Design review of the part shown in the three views and the two pictorial views. Dimensions are in mm from the part's minimum x, y and z. Coordinates: 2 decimals unless noted, no trailing zeros. Write each loop counter-clockwise with the first axis right and the second up, starting at its lowest first coordinate (ties: lowest second). Pieces come first, ordered by that corner, then holes. Notation, with made-up numbers: M -10.75,30.25 L 24.25,30.25 A17 cw 24.25,35.25 Z; hole C -6,63 d8. An arc over 180 degrees is marked long. Answer as a JSON object with one key per item and string values.
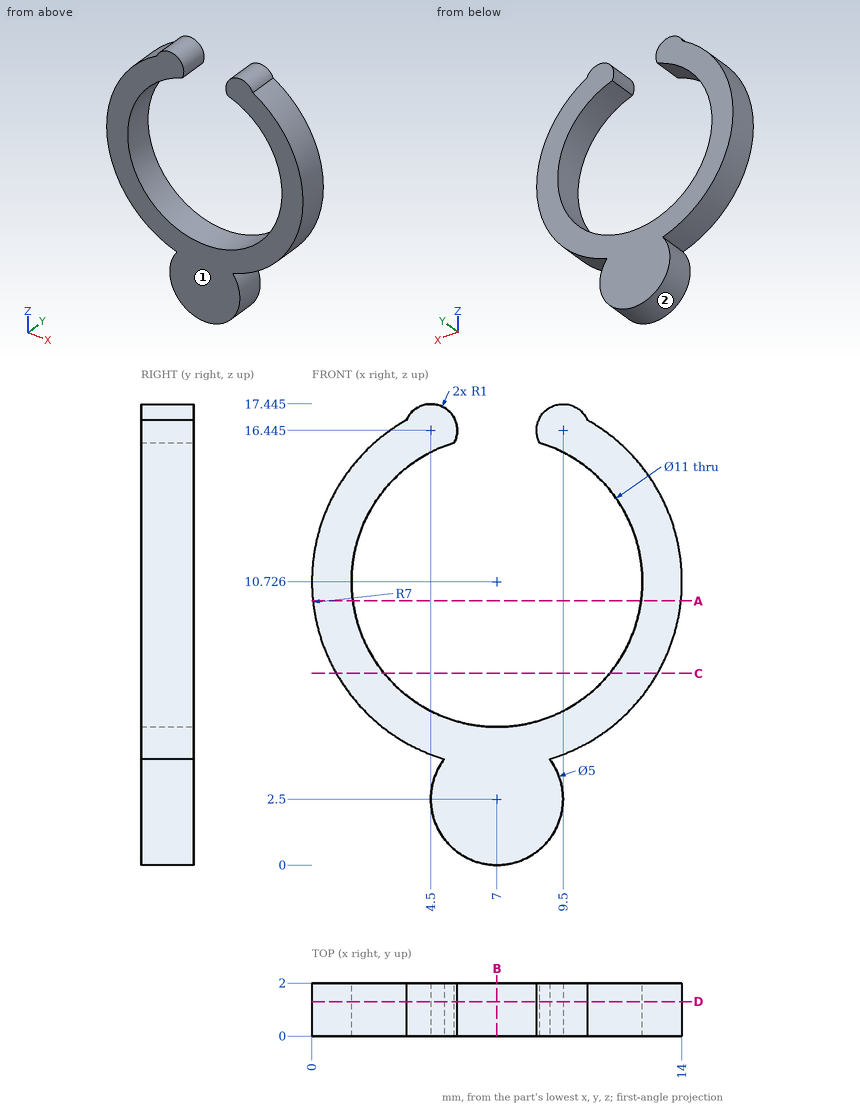
(1) Add section A-A on z = 10. Give the boundary of the cut face in (x, y).
Results list:
{"outline": "M 0.04,0 L 1.55,0 L 1.55,2 L 0.04,2 Z; M 12.45,0 L 13.96,0 L 13.96,2 L 12.45,2 Z"}
(2) For pin 1 Ø1 at (y, z) = (1.5, 6.5) entering from -X (1 decimal); pin 2 Ø8 at (x, z) = (12, 15.5) entering from -Y, all flat-tipped, find the tip position at first contact; note any pin that passes through.
Results list:
{"pin 1": "x = 1.1", "pin 2": "y = 0"}
(3) Draft analysis for pull direction Z (two halves, no side actions). For the marked faces 1 and 2, state which applies: released by +Z, released by -Z, zero draft, split by the parting line, or undercut.
Results list:
{"face 1": "zero draft", "face 2": "undercut"}
(4) Add section D-D on y = 1.3. Give the boundary of the cut face in (x, z) (1 decimal).
Results list:
{"outline": "M 3.6,16.8 A7 ccw 5,4 A2.5 ccw long 9,4 A7 ccw 10.4,16.8 A1 ccw long 8.6,16 A5.5 cw long 5.4,16 A1 ccw long Z"}
(5) Add section C-C on z = 7.25. Give the boundary of the cut face in (x, y).
Results list:
{"outline": "M 0.92,0 L 2.74,0 L 2.74,2 L 0.92,2 Z; M 11.26,0 L 13.08,0 L 13.08,2 L 11.26,2 Z"}
(6) Wall thickness on line 1 along X through (y, z) = (0.9, 10.5) (1 decimal); line 2 along Z through (x, y) = (4.75, 1.1) (1 decimal); line 3 along X through (y, z) = (1.55, 14): over which ranges is each line inside the solid? List them lowest first. Write a range as from..to.
Results list:
{"line 1": "0..1.5, 12.5..14", "line 2": "1.4..3.6, 4.1..5.7, 15.7..17.4", "line 3": "0.81..2.58, 11.42..13.19"}
(7) Add section B-B on x = 7. Give the boundary of the cut face in (y, z).
Results list:
{"outline": "M 0,0 L 2,0 L 2,5.23 L 0,5.23 Z"}
